from build123d import *

# Parameters (mm, degrees)
BOSS_EXTRUDE1_DEPTH = 2.54
SKETCH3_R           = 14.2875
CUT_EXTRUDE1_DEPTH  = 68.843323924
FILLET1_R           = 2.54


with BuildPart() as part:
    # Sketch1 → Boss-Extrude1 (new body)
    with BuildSketch(Plane(origin=(0, 0, 0), x_dir=(0, 0, -1), z_dir=(1, 0, 0))):
        with BuildLine():
            Line((-63.5, -23.749), (63.5, -23.749))
            Line((63.5, -23.749), (63.5, 1.651))
            Line((63.5, 1.651), (5.238797024, 18.315499058))
            ThreePointArc((5.238797024, 18.315499058), (0, 19.05), (-5.238797024, 18.315499058))
            Line((-5.238797024, 18.315499058), (-63.5, 1.651))
            Line((-63.5, 1.651), (-63.5, -23.749))
        make_face()
    extrude(amount=BOSS_EXTRUDE1_DEPTH)

    # Sketch3 → Cut-Extrude1 (cut, through all)
    with BuildSketch(Plane.ZY):
        Circle(SKETCH3_R)
        with BuildLine():
            Line((-53.975, -8.8773), (-47.625, -8.8773))
            ThreePointArc((-47.625, -8.8773), (-45.4533, -11.049), (-47.625, -13.2207))
            Line((-47.625, -13.2207), (-53.975, -13.2207))
            ThreePointArc((-53.975, -13.2207), (-56.1467, -11.049), (-53.975, -8.8773))
        make_face()
        with BuildLine():
            Line((-28.575, -8.8773), (-22.225, -8.8773))
            ThreePointArc((-22.225, -8.8773), (-20.0533, -11.049), (-22.225, -13.2207))
            Line((-22.225, -13.2207), (-28.575, -13.2207))
            ThreePointArc((-28.575, -13.2207), (-30.7467, -11.049), (-28.575, -8.8773))
        make_face()
        with BuildLine():
            Line((22.225, -8.8773), (28.575, -8.8773))
            ThreePointArc((28.575, -8.8773), (30.7467, -11.049), (28.575, -13.2207))
            Line((28.575, -13.2207), (22.225, -13.2207))
            ThreePointArc((22.225, -13.2207), (20.0533, -11.049), (22.225, -8.8773))
        make_face()
        with BuildLine():
            Line((47.625, -8.8773), (53.975, -8.8773))
            ThreePointArc((53.975, -8.8773), (56.1467, -11.049), (53.975, -13.2207))
            Line((53.975, -13.2207), (47.625, -13.2207))
            ThreePointArc((47.625, -13.2207), (45.4533, -11.049), (47.625, -8.8773))
        make_face()
    extrude(amount=-CUT_EXTRUDE1_DEPTH, mode=Mode.SUBTRACT)

    # Fillet1
    fillet1_edges = [part.edges().sort_by_distance(p)[0] for p in [
        (1.27, -23.749, 63.5),
        (1.27, 1.651, 63.5),
        (1.27, 1.651, -63.5),
        (1.27, -23.749, -63.5),
    ]]
    fillet(fillet1_edges, radius=FILLET1_R)


solid = part.part
Geometry: final body of the model. Coordinates: model frame, mm. A direction names the side the tool comes from. Round coordinates to 2 decimals unless told otherwise and drop trailing zeros. Order: outer loops, then holes, each group sorted by start corner. A loop starts at its lowest first (then second) coordinate and runs counter-clockwise, first axis right, second up.
Q1. Access query for faces 1 (the face through (1, -8.877, -25)), 2 (the face through (1.25, 19.05, -0.07)). Directions: +Z, -Z, +X, -X, +Y, -Y. A direction counts if a zero-diameter tool reaches every point of the face in a straight line with its end or side. Return the directions, or none.
Result sheet:
face 1: +X, -X
face 2: +X, -X, +Y
Q2. Pin query (flat end, axial travel): pin 1 (8 mm diameter, centred on y = 11, z = 44.5, fed in from +X); pin 2 (0.8 mm diameter, centred on x = 1, z = -51, fed in from +Y); pin 3 (0.8 mm diameter, centred on x = 1.5, z = -24, fed in from +Y); pin 4 (1.3 mm diameter, centred on x = 1, z = 26, fed in from +Y). Return the tip coordinate at first contact, or that it passes through.
Result sheet:
pin 1: stops at x = 2.54
pin 2: stops at y = 5.34
pin 3: stops at y = 13.06
pin 4: stops at y = 12.56
Q3. Section B-B, the plane y = 6. Output: boundary loops of the cut face in (x, z), and give its area (3 significant figures).
Result sheet:
outline: (0, -48.3) - (2.54, -48.3) - (2.54, -12.97) - (0, -12.97) - close; (0, 12.97) - (2.54, 12.97) - (2.54, 48.3) - (0, 48.3) - close
area: 179 mm2
Q4. Section A-A, the plane z = 0. Output: boundary loops of the cut face in (x, y).
Result sheet:
outline: (0, -23.75) - (2.54, -23.75) - (2.54, -14.29) - (0, -14.29) - close; (0, 14.29) - (2.54, 14.29) - (2.54, 19.05) - (0, 19.05) - close
Q5. Mould query, pull axis Z, two halves, no side actions, for faces 3 (the face through (1, -11, -63.5)), 4 (the face through (1.252, -11.001, 30.746)), 5 (the face through (1.29, 1.25, 63)), 6 (the face through (0, -16, 1)). Classes: released by +Z, released by -Z, zero draft, split by the parting line, or undercut.
Result sheet:
face 3: released by -Z
face 4: undercut
face 5: released by +Z
face 6: zero draft
Q6. Section D-D, the plane y = 16.5. Output: boundary loops of the cut face in (x, z), and give its area (3 significant figures).
Result sheet:
outline: (0, -11.59) - (2.54, -11.59) - (2.54, 11.59) - (0, 11.59) - close
area: 58.9 mm2
Q7. Section C-C, the plane x = 2.1. Give the number of separate pieces and of enclosed holes in the cut face, and give its area (3 significant figures).
Result sheet:
separate pieces: 1
enclosed holes: 5
area: 3,560 mm2
Q8. Material intervals for probe 1 along Y at (x, z) = (1.95, 0); probe 2 along Y at (x, z) = (0.6, 53.5); probe 3 along Z at (x, y) = (1.5, -3.5), sorted ascending.
Result sheet:
probe 1: y = -23.75 to -14.29, 14.29 to 19.05
probe 2: y = -23.75 to -13.22, -8.88 to 4.51
probe 3: z = -63.5 to -13.85, 13.85 to 63.5
